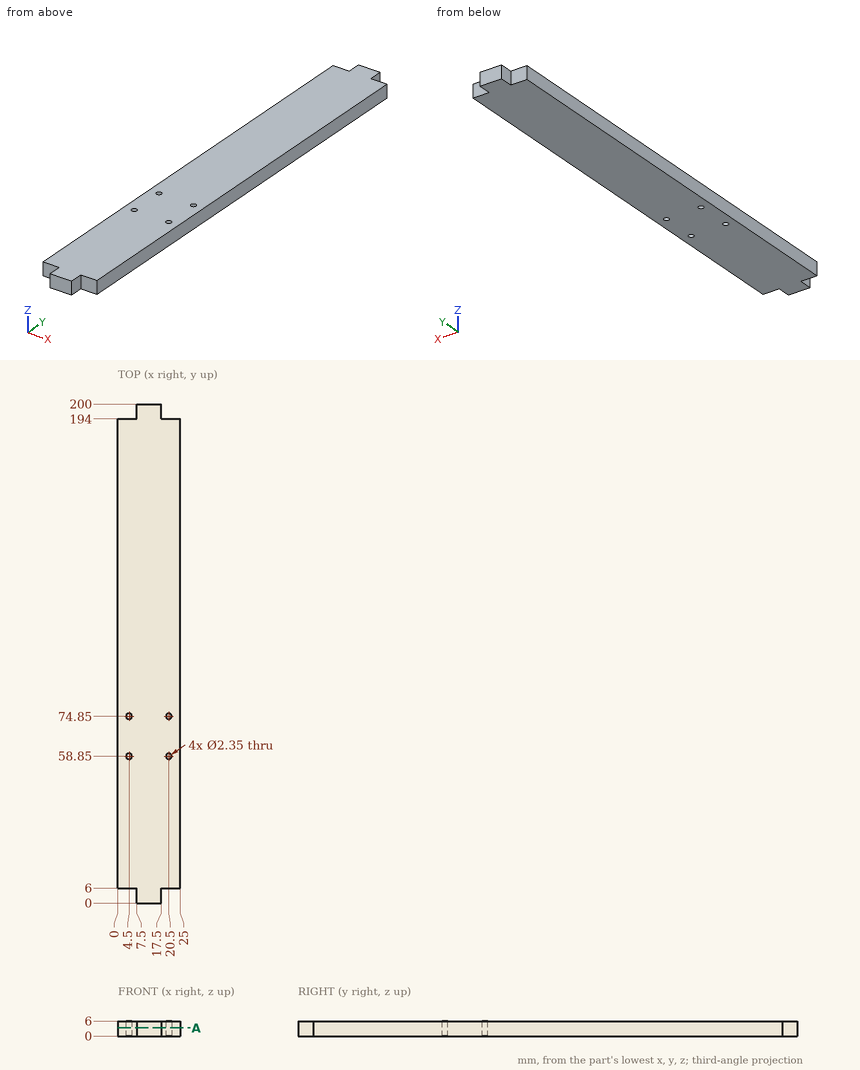
Could you check a few things on this drawing? It's one solid part, dimensions in mm from its lowest x, y, z. Coordinates: 2 decimals unless noted, no trailing zeros. Loops run counter-clockwise (first coordinate to the right, second up) from the corner with the lowest first, then second, coordinate; pieces in that order, holes last.
1. For P1, Ø3, axis at x = 5, z = 3, coming from the -Y side; P2, Ø1.5, axis at y = 161.5, z = 2, coming from the -X side; P3, Ø1.8, axis at y = 4, z = 2, coming from the +X side; P4, Ø1.8, axis at x = 21.5, z = 4, coming from the +Y side, each with a flat end and sliding along its axis, tell me the tip position at first contact or that it passes through.
2. I need wall thicknesses on L1, parallel to Y at x = 4.5, z = 4.2 (3 decimals); L2, parallel to X at y = 58.85, z = 2.05 (3 decimals); L3, parallel to Y at x = 21.5, z = 1.35. Which ranges of each line are inside material? Lowest first, please.
3. Imagine slicing it at A-A (z = 3.3). Please give me the cut outline in (x, y) (3 decimals).
Computed values:
1. P1: stops at y = 6
1. P2: stops at x = 0
1. P3: stops at x = 17.5
1. P4: stops at y = 194
2. L1: y = 6 to 57.675, 60.025 to 73.675, 76.025 to 194
2. L2: x = 0 to 3.325, 5.675 to 19.325, 21.675 to 25
2. L3: y = 6 to 58.23, 59.47 to 74.23, 75.47 to 194
3. outline: (0, 6) - (7.5, 6) - (7.5, 0) - (17.5, 0) - (17.5, 6) - (25, 6) - (25, 194) - (17.5, 194) - (17.5, 200) - (7.5, 200) - (7.5, 194) - (0, 194) - close; hole circle Ø2.35 at (4.5, 58.85); hole circle Ø2.35 at (4.5, 74.85); hole circle Ø2.35 at (20.5, 58.85); hole circle Ø2.35 at (20.5, 74.85)
